CAD build for the part. Positions are in the model's coordinates, mm. Face numbers are marked on the shaded views. A direction names the side the tool comes from. Coordinates: 2 decimals unless noted, no trailing zeros. Write each loop counter-clockwise with the first axis right and the second up, starting at its lowest first coordinate (ties: lowest second). Pieces come first, ordered by that corner, then holes.
```python
from build123d import *

# Parameters (mm, degrees)
SKETCH_1_R          = 5
SKETCH_1_R_2        = 1.225
SKETCH_1_R_3        = 1.025
EXTRUDE_1_DEPTH     = 60
SKETCH_2_W          = 57.132931415
SKETCH_2_H          = 51.5
CUT_EXTRUDE_1_DEPTH = 66
CUT_EXTRUDE_START   = -60.33903683
CUT_EXTRUDE_3_DEPTH = 60.33903683
SKETCH_6_R          = 1.25
CUT_EXTRUDE_4_DEPTH = 10


with BuildPart() as part:
    # 스케치1 → 보스-돌출1 (new body)
    with BuildSketch(Plane.XY):
        with BuildLine():
            Line((11.674013781, 7.727703555), (-14, 46.512678751))
            Line((-14, 46.512678751), (-47.132931415, 46.512678751))
            Line((-47.132931415, 46.512678751), (-47.132931415, 14.921692086))
            Line((-47.132931415, 14.921692086), (-11, -8.660254038))
            ThreePointArc((-11, -8.660254038), (8.200906179, -11.346591463), (11.674013781, 7.727703555))
        make_face()
        Circle(SKETCH_1_R, mode=Mode.SUBTRACT)
        with Locations((0, 8)):
            Circle(SKETCH_1_R_2, mode=Mode.SUBTRACT)
        with Locations((0, 11)):
            Circle(SKETCH_1_R_2, mode=Mode.SUBTRACT)
        with Locations((7.778174593, 7.778174593)):
            Circle(SKETCH_1_R_2, mode=Mode.SUBTRACT)
        with Locations((8, 0)):
            Circle(SKETCH_1_R_2, mode=Mode.SUBTRACT)
        with Locations((11, 0)):
            Circle(SKETCH_1_R_2, mode=Mode.SUBTRACT)
        with Locations((7.778174593, -7.778174593)):
            Circle(SKETCH_1_R_2, mode=Mode.SUBTRACT)
        with Locations((0, -8)):
            Circle(SKETCH_1_R_2, mode=Mode.SUBTRACT)
        with Locations((0, -11)):
            Circle(SKETCH_1_R_2, mode=Mode.SUBTRACT)
        with Locations((-7.778174593, -7.778174593)):
            Circle(SKETCH_1_R_2, mode=Mode.SUBTRACT)
        with Locations((-8, 0)):
            Circle(SKETCH_1_R_3, mode=Mode.SUBTRACT)
        with Locations((-11, 0)):
            Circle(SKETCH_1_R_2, mode=Mode.SUBTRACT)
        with Locations((-7.778174593, 7.778174593)):
            Circle(SKETCH_1_R_2, mode=Mode.SUBTRACT)
    extrude(amount=EXTRUDE_1_DEPTH)

    # 스케치2 → 컷-돌출1 (cut)
    with BuildSketch(Plane(origin=(0, 46.512678751, 0), x_dir=(1, 0, 0), z_dir=(0, 1, 0))):
        with Locations((-14.566465708, -29.75)):
            Rectangle(SKETCH_2_W, SKETCH_2_H)
    extrude(amount=-CUT_EXTRUDE_1_DEPTH, mode=Mode.SUBTRACT)

    # 스케치4 → 컷-돌출3 (cut)
    with BuildSketch(Plane.XY.offset(60).offset(CUT_EXTRUDE_START)):
        with BuildLine():
            Line((-5, 0), (-5, -13.076696831))
            ThreePointArc((-5, -13.076696831), (0, -14), (5, -13.076696831))
            Line((5, -13.076696831), (5, 0))
            Line((5, 0), (-5, 0))
        make_face()
    extrude(amount=CUT_EXTRUDE_3_DEPTH, mode=Mode.SUBTRACT)

    # 스케치6 → 컷-돌출4 (cut)
    with BuildSketch(Plane.ZY.offset(47.132931415)):
        with Locations(Location((30, 30.717185419, 0), (0, 0, 270))):
            Circle(SKETCH_6_R)
        with Locations(Location((40, 30.717185419, 0), (0, 0, 270))):
            Circle(SKETCH_6_R)
        with Locations(Location((20, 30.717185419, 0), (0, 0, 270))):
            Circle(SKETCH_6_R)
        with Locations(Location((20, 40.717185419, 0), (0, 0, 270))):
            Circle(SKETCH_6_R)
        with Locations(Location((30, 40.717185419, 0), (0, 0, 270))):
            Circle(SKETCH_6_R)
        with Locations(Location((40, 40.717185419, 0), (0, 0, 270))):
            Circle(SKETCH_6_R)
        with Locations(Location((20, 20.717185419, 0), (0, 0, 270))):
            Circle(SKETCH_6_R)
        with Locations(Location((30, 20.717185419, 0), (0, 0, 270))):
            Circle(SKETCH_6_R)
        with Locations(Location((40, 20.717185419, 0), (0, 0, 270))):
            Circle(SKETCH_6_R)
    extrude(amount=-CUT_EXTRUDE_4_DEPTH, mode=Mode.SUBTRACT)


solid = part.part
```
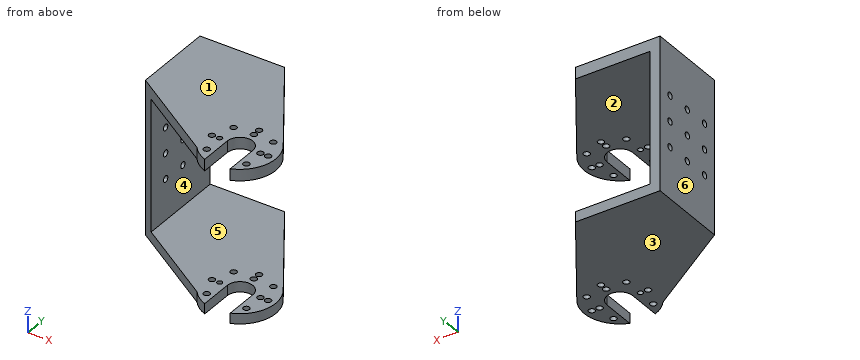
Item 1: Two-plate mould, pull along Z, no slides. Class the marked faces 1, 2, 3 and 4: +Z half, -Z half, draft (parallel to the pull), parting line (faces both ways), or undercut.
Item 2: Saw through at B-B, the plane x = -29. Write the cut outline in (y, z).
Item 3: Saw through at A-A, the plane z = 30. Write the cut outline in (x, y).
Item 4: Which spindle directions (+Z, -Z, +X, -X, +Y, -Y) get a long thin tool onto all of the face, cutting with end or side? Do the marked faces 5 and 6. Say none if no direction does.
Item 5: Saw through at C-C, the plane y = 11. Write the cut outline in (x, z) (3 decimals), and give its area (3 significant figures).
Item 6: Saw through at D-D, the plane x = -8. State how many separate pieces and enclosed holes the cut face has, and give its area (3 significant figures).
Item 7: Wall check: line 1 along Z through (x, y) = (-11, 33); line 2 along X through (y, z) = (0, 58.3) (3 decimals); line 3 along X through (y, z) = (35.5, 29.5). Give the ranges that are in metal, low to high.
Item 8: Flat gauge pins, fed straight in: pin 1 Ø3 at (y, z) = (20.72, 30) entering from +X; pin 2 Ø10 at (y, z) = (2.5, 53) entering from -X. Where does each tip first touch, or does it go through?
Working result:
1. face 1: +Z half
1. face 2: undercut
1. face 3: -Z half
1. face 4: undercut
2. outline: (3.09, 0) - (46.51, 0) - (46.51, 4) - (3.09, 4) - close; (3.09, 55.5) - (46.51, 55.5) - (46.51, 60) - (3.09, 60) - close
3. outline: (-47.13, 14.92) - (-43.13, 12.31) - (-43.13, 19.47) - (-47.13, 19.47) - close; (-47.13, 21.97) - (-43.13, 21.97) - (-43.13, 29.47) - (-47.13, 29.47) - close; (-47.13, 31.97) - (-43.13, 31.97) - (-43.13, 39.47) - (-47.13, 39.47) - close; (-47.13, 41.97) - (-43.13, 41.97) - (-43.13, 46.51) - (-47.13, 46.51) - close
4. face 5: +X, +Y, -Y
4. face 6: +Z, -Z, -X, +Y, -Y
5. outline: (-41.124, 0) - (-1.225, 0) - (-1.225, 4) - (-41.124, 4) - close; (-41.124, 55.5) - (-1.225, 55.5) - (-1.225, 60) - (-41.124, 60) - close; (1.225, 0) - (9.508, 0) - (9.508, 4) - (1.225, 4) - close; (1.225, 55.5) - (9.508, 55.5) - (9.508, 60) - (1.225, 60) - close
5. area: 410 mm2
6. separate pieces: 8
6. enclosed holes: 0
6. area: 358 mm2
7. line 1: z = 0 to 4, 55.5 to 60
7. line 2: x = -24.269 to -12.225, -9.775 to -9.025, -6.975 to -5, 5 to 6.775, 9.225 to 9.775, 12.225 to 14
7. line 3: x = -47.13 to -43.13
8. pin 1: stops at x = -43.13
8. pin 2: stops at x = -34.73
